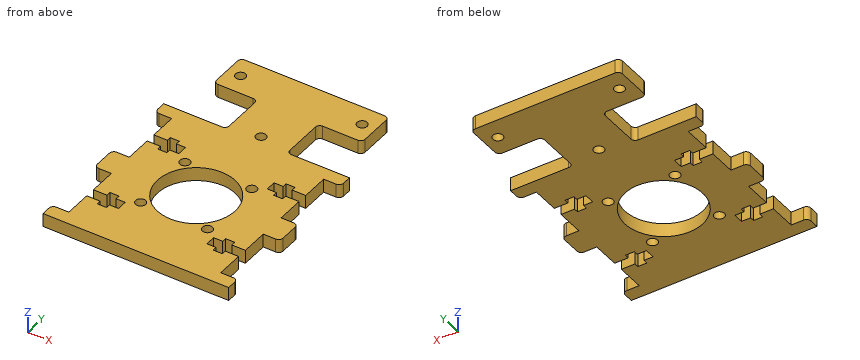
from build123d import *

# Parameters (mm, degrees)
SKETCH_1_R      = 1.5
SKETCH_1_R_2    = 11.5
EXTRUDE_1_DEPTH = 4
FILLET_1_R      = 1.3


with BuildPart() as part:
    # 草图1 → 凸台-拉伸1 (new body)
    with BuildSketch(Plane.XY):
        Polygon((22.5, -27), (-22.5, -27), (-27.5, -27), (-27.5, -23), (-22.5, -23), (-22.5, -15), (-18.5, -15), (-18.5, -16.3), (-15.8, -16.3), (-15.8, -15), (-13.1, -15), (-13.1, -12), (-15.8, -12), (-15.8, -10.7), (-18.5, -10.7), (-18.5, -12), (-22.5, -12), (-22.5, -4), (-27.5, -4), (-27.5, 4), (-22.5, 4), (-22.5, 12), (-18.5, 12), (-18.5, 10.7), (-15.8, 10.7), (-15.8, 12), (-13.1, 12), (-13.1, 15), (-15.8, 15), (-15.8, 16.3), (-18.5, 16.3), (-18.5, 15), (-22.5, 15), (-22.5, 23), (-27.5, 23), (-27.5, 27), (-22.5, 27), (-9, 27), (-9, 41), (-22, 41), (-22, 53), (22, 53), (22, 41), (9, 41), (9, 27), (22.5, 27), (27.5, 27), (27.5, 23), (22.5, 23), (22.5, 15), (18.5, 15), (18.5, 16.3), (15.8, 16.3), (15.8, 15), (13.1, 15), (13.1, 12), (15.8, 12), (15.8, 10.7), (18.5, 10.7), (18.5, 12), (22.5, 12), (22.5, 4), (27.5, 4), (27.5, -4), (22.5, -4), (22.5, -12), (18.5, -12), (18.5, -10.7), (15.8, -10.7), (15.8, -12), (13.1, -12), (13.1, -15), (15.8, -15), (15.8, -16.3), (18.5, -16.3), (18.5, -15), (22.5, -15), (22.5, -23), (27.5, -23), (27.5, -27), align=None)
        with Locations((9.899494937, 9.899494937)):
            Circle(SKETCH_1_R, mode=Mode.SUBTRACT)
        Circle(SKETCH_1_R_2, mode=Mode.SUBTRACT)
        with Locations((9.899494937, -9.899494937)):
            Circle(SKETCH_1_R, mode=Mode.SUBTRACT)
        with Locations((-9.899494937, -9.899494937)):
            Circle(SKETCH_1_R, mode=Mode.SUBTRACT)
        with Locations((-9.899494937, 9.899494937)):
            Circle(SKETCH_1_R, mode=Mode.SUBTRACT)
        with Locations((-18, 47)):
            Circle(SKETCH_1_R, mode=Mode.SUBTRACT)
        with Locations((18, 47)):
            Circle(SKETCH_1_R, mode=Mode.SUBTRACT)
        with Locations((0, 29)):
            Circle(SKETCH_1_R, mode=Mode.SUBTRACT)
    extrude(amount=EXTRUDE_1_DEPTH)

    # 圆角1
    fillet_1_edges = [part.edges().sort_by_distance(p)[0] for p in [
        (-9, 27, 2),
        (-9, 41, 2),
        (-22, 41, 2),
        (-22, 53, 2),
        (22, 53, 2),
        (22, 41, 2),
        (9, 41, 2),
        (9, 27, 2),
        (27.5, 23, 2),
        (27.5, 4, 2),
        (27.5, -4, 2),
        (27.5, -23, 2),
        (-27.5, -23, 2),
        (-27.5, -4, 2),
        (-27.5, 4, 2),
        (-27.5, 23, 2),
    ]]
    fillet(fillet_1_edges, radius=FILLET_1_R)


solid = part.part
The listing builds one solid part. Answer for the finished solid, in the listing's coordinates (mm). Give positions to 0.01 mm unless a question says otherwise; leave off trailing zeros. Order: outer loops, then holes, each group sorted by start corner. A loop starts at its lowest first (then second) coordinate and runs counter-clockwise, first axis right, second up. Notation, with made-up numbers: (75, 66) -> (106, 66) arc R21 cw to (106, 87) -> close; hole circle Ø8 at (24.25, 65). An arc over 180 degrees is marked (long way). Put each result on its own line as item: value.
Item 1: Given P1, Ø12, axis at x = -9.5, y = -4, coming from the -Z side; P2, Ø1, axis at y = 15.5, z = 2.5, coming from the -X side; P3, Ø1.1, axis at x = 24.5, z = 2, coming from the +Y side, each flat-ended and moving along its own axis, determine where each tip first touches the part or whether it passes through.
Established:
P1: stops at z = 0
P2: stops at x = -22.5
P3: stops at y = 27
Item 2: A cutting plane is placed at D-D on y = -18.5. Give the vertices of the cut face in (x, z).
Established:
outline: (-22.5, 0) -> (22.5, 0) -> (22.5, 4) -> (-22.5, 4) -> close
Item 3: A cutting plane is placed at C-C on y = 0. Give the vertices of the cut face in (x, z).
Established:
outline: (-27.5, 0) -> (-11.5, 0) -> (-11.5, 4) -> (-27.5, 4) -> close; (11.5, 0) -> (27.5, 0) -> (27.5, 4) -> (11.5, 4) -> close
Item 4: A cutting plane is placed at A-A on x = 0. Give the vertices of the cut face in (y, z), plus the area to 3 significant figures.
Established:
outline: (-27, 0) -> (-11.5, 0) -> (-11.5, 4) -> (-27, 4) -> close; (11.5, 0) -> (27.5, 0) -> (27.5, 4) -> (11.5, 4) -> close; (30.5, 0) -> (53, 0) -> (53, 4) -> (30.5, 4) -> close
area: 216 mm^2
Item 5: Straight lines are drawn through the part: line 1 (Y direction, x = -15, z = 2.85); line 2 (Y direction, x = 0, z = 2.8); line 3 (Y direction, x = 24, z = 2.8). For each, find the intervals that lie inside material, in ascending order.
Established:
line 1: y = -27 to -15, -12 to 12, 15 to 27, 41 to 53
line 2: y = -27 to -11.5, 11.5 to 27.5, 30.5 to 53
line 3: y = -27 to -23, -4 to 4, 23 to 27
Item 6: A cutting plane is placed at B-B on y = 47. Give the vertices of the cut face in (x, z).
Established:
outline: (-22, 0) -> (-19.5, 0) -> (-19.5, 4) -> (-22, 4) -> close; (-16.5, 0) -> (16.5, 0) -> (16.5, 4) -> (-16.5, 4) -> close; (19.5, 0) -> (22, 0) -> (22, 4) -> (19.5, 4) -> close
